from build123d import *

# Parameters (mm, degrees)
SKETCH1_W               = 15
SKETCH1_H               = 15
SKETCH1_W_2             = 13
SKETCH1_H_2             = 13
SKETCH1_R               = 2
BOSS_EXTRUDE1_DEPTH     = 7.5
CUT_EXTRUDE1_DEPTH      = 13.990381057
CUT_EXTRUDE1_DEPTH_BACK = 13.990381057
CUT_EXTRUDE2_DEPTH      = 13.99038123
CUT_EXTRUDE2_DEPTH_BACK = 13.99038123
SKETCH1_3_W             = 13
SKETCH1_3_H             = 13
SKETCH1_3_R             = 2
CUT_EXTRUDE3_DEPTH      = 5


with BuildPart() as part:
    # Sketch1 → Boss-Extrude1 (new body)
    # profile 1 of 3: a face of its own
    with BuildSketch(Plane(origin=(0, 0, 0), x_dir=(1, 0, 0), z_dir=(0, 1, 0))):
        Rectangle(SKETCH1_W, SKETCH1_H)
        Rectangle(SKETCH1_W_2, SKETCH1_H_2, mode=Mode.SUBTRACT)
    # profile 2 of 3: a face of its own
    with BuildSketch(Plane(origin=(0, 0, 0), x_dir=(1, 0, 0), z_dir=(0, 1, 0))):
        Rectangle(SKETCH1_W_2, SKETCH1_H_2)
        Circle(SKETCH1_R, mode=Mode.SUBTRACT)
    # profile 3 of 3: a face of its own
    with BuildSketch(Plane(origin=(0, 0, 0), x_dir=(1, 0, 0), z_dir=(0, 1, 0))):
        Circle(SKETCH1_R)
    extrude(amount=BOSS_EXTRUDE1_DEPTH)

    # Sketch2 → Cut-Extrude1 (cut, two sides: drawn at the far end of the back side and taken through both)
    with BuildSketch(Plane.XY.offset(-CUT_EXTRUDE1_DEPTH_BACK)):
        with BuildLine():
            Line((-10, 12), (-10, 0))
            Line((-10, 0), (-7.5, 0))
            add(Edge.make_bspline(
                [(0, 12), (-7.5, 12), (-7.5, 0)],
                knots=[0, 0, 0, 1.570796327, 1.570796327, 1.570796327], degree=2, weights=[1, 0.707106781, 1]))
            Line((0, 12), (-10, 12))
        make_face()
        with BuildLine():
            add(Edge.make_bspline(
                [(7.5, 0), (7.5, 12), (0, 12)],
                knots=[4.71238898, 4.71238898, 4.71238898, 6.283185307, 6.283185307, 6.283185307], degree=2, weights=[1, 0.707106781, 1]))
            Line((7.5, 0), (10, 0))
            Line((10, 0), (10, 12))
            Line((10, 12), (0, 12))
        make_face()
    extrude(amount=CUT_EXTRUDE1_DEPTH + CUT_EXTRUDE1_DEPTH_BACK, mode=Mode.SUBTRACT)

    # Sketch3 → Cut-Extrude2 (cut, two sides: drawn at the far end of the back side and taken through both)
    with BuildSketch(Plane(origin=(0, 0, 0), x_dir=(0, 0, -1), z_dir=(1, 0, 0)).offset(-CUT_EXTRUDE2_DEPTH_BACK)):
        with BuildLine():
            Line((7.5, 0), (10, 0))
            Line((10, 0), (10, 12))
            Line((10, 12), (0, 12))
            add(Edge.make_bspline(
                [(7.5, 0), (7.5, 12), (0, 12)],
                knots=[1.570796327, 1.570796327, 1.570796327, 3.141592654, 3.141592654, 3.141592654], degree=2, weights=[1, 0.707106781, 1]))
        make_face()
        with BuildLine():
            Line((-10, 0), (-7.5, 0))
            add(Edge.make_bspline(
                [(0, 12), (-7.5, 12), (-7.5, 0)],
                knots=[3.141592654, 3.141592654, 3.141592654, 4.71238898, 4.71238898, 4.71238898], degree=2, weights=[1, 0.707106781, 1]))
            Line((0, 12), (-10, 12))
            Line((-10, 12), (-10, 0))
        make_face()
    extrude(amount=CUT_EXTRUDE2_DEPTH + CUT_EXTRUDE2_DEPTH_BACK, mode=Mode.SUBTRACT)

    # Sketch1_3 → Cut-Extrude3 (cut)
    with BuildSketch(Plane(origin=(0, 0, 0), x_dir=(1, 0, 0), z_dir=(0, 1, 0))):
        Rectangle(SKETCH1_3_W, SKETCH1_3_H)
        with Locations(Location((0, 0, 0), (0, 0, 270))):
            Circle(SKETCH1_3_R, mode=Mode.SUBTRACT)
    extrude(amount=CUT_EXTRUDE3_DEPTH, mode=Mode.SUBTRACT)


solid = part.part
Can you work these out from the model? Positions are in its coordinate system, mm. A direction names the side the tool comes from. Coordinates: 2 decimals unless noted, no trailing zeros. Put each result on its own line as item: value. Start each with the question number.
Item 1: Suppose I cut it at A-A (y = 2.5). State how many separate pieces and enclosed holes the cut face has, and give its area (3 significant figures).
Item 2: If I drill on line 1 along X through (y, z) = (2.25, 0); line 2 along Y through (x, z) = (-3.5, 0.5); line 3 along Z through (x, y) = (5.75, 6), over which ranges is the centre line in solid material (lowest first)?
Item 3: Which directions (+Z, -Z, +X, -X, +Y, -Y) give clear straight access to the entire face, cutting with the end or side of a thin tool? Please do faces 1 (the face through (0, 0, 0)), 2 (the face through (-6.5, 2, 0)).
Item 4: If we mould it in two halves opening along X, with no side actions, what happens to faces 3 (the face through (6.5, 2, 0)), 4 (the face through (0, 7.5, 0)), 5 (the face through (-2, 5, -2))? For each: +X half, -X half, draft (parallel to the pull), parting line (faces both ways), or undercut.
Item 5: For pin 1 (4 mm diameter, centred on y = 5.5, z = -2.5, fed in from -X); pin 2 (2 mm diameter, centred on x = 5.5, y = 6.5, fed in from -Z); pin 3 (1 mm diameter, centred on y = 2.5, z = -5, fed in from +X), each with a flat end and sliding along its axis, tell me the tip position at first contact or that it passes through.
Here are the results:
1. separate pieces: 2
1. enclosed holes: 1
1. area: 58.8 mm²
2. line 1: -7.37 to -6.5, -2 to 2, 6.5 to 7.37
2. line 2: 5 to 7.5
2. line 3: -6.5 to 6.5
3. face 1: +Z, -Z, +X, -X, -Y
3. face 2: -Y
4. face 3: undercut
4. face 4: draft
4. face 5: undercut
5. pin 1: x = -7.17
5. pin 2: z = -6.67
5. pin 3: x = 7.4
